Autodesk Fusion 360 part; units mm, degrees
sketch "Sketch1" plane through (0, 0, 0) normal (0, 0, 1) x (1, 0, 0)
  circle A0 centre (0, 0) radius 1.75
  circle A1 centre (0, 0) radius 5.25
  dimension "d1" = 3.5
  dimension "d2" = 3.5
extrude "Extrude1" add sketch "Sketch1" along normal blind 5
chamfer "Chamfer1" distance 1 angle 45 4 edges at (-1.6316, 0.6328, 5) (-4.8947, -1.8985, 5) (-4.8947, -1.8985, 0) (-1.6316, 0.6328, 0)
fillet "Fillet1" radius 1.25 4 edges at (-4.8947, -1.8985, 4) (-4.8947, 1.8985, 1) (-1.6316, 0.6328, 4) (-1.6316, -0.6328, 1)
fillet "Fillet2" radius 1.4 4 edges at (-3.9624, -1.5369, 0) (-2.5639, 0.9944, 0) (-2.5639, -0.9944, 5) (-3.9624, 1.5369, 5)
Geometry check sheet. Reference: the model listing, model coordinates, mm. Give positions to 0.01 mm unless a question says otherwise; leave off trailing zeros. Loops run counter-clockwise (first coordinate to the right, second up) from the corner with the lowest first, then second, coordinate; pieces in that order, holes last. Notation, with made-up numbers: M 64.25,65 L 85.25,65 A23 ccw 85.25,100 Z; hole C 26,39 d5. An arc over 180 degrees is marked long. Answer as a JSON object with one key per item and string values. Group by question number.
Item 1: Mould release check, pull along X, two halves, no side actions. Record for faces 1 (the cylindrical face through (1.617, 0.67, 2.486)), 2 (the cylindrical face through (5, -1.6, 2.5)): pulls with the +X half, pulls with the -X half, needs draft (parallel to the pull), parting line crosses it, or undercut.
Item 2: Gauge pin test, flat ends, axial feed: pin 1 (2 mm diameter, centred on x = 1.5, z = 2, fed in from -Y); pin 2 (2 mm diameter, centred on y = 4, z = 4, fed in from -X); pin 3 (1.5 mm diameter, centred on x = 2.5, z = 4, fed in from -Y). Record the tip position at first contact, or that the pin passes through.
Item 3: Material ranges on L1, parallel to Y at x = 0, z = 2.85; L2, parallel to X at y = -0.25, z = 3.75, recorded low to high.
Item 4: Sectioned sample at A-A on z = 2.45. Record the boundary of the cut face in (x, y), plus the area to 3 significant figures.
Findings below:
{
 "1": {"face 1": "undercut", "face 2": "parting line crosses it"},
 "2": {"pin 1": "y = -5.23", "pin 2": "x = -4.25", "pin 3": "y = -4.91"},
 "3": {"L1": "-5.25 to -1.75, 1.75 to 5.25", "L2": "-5.21 to -1.76, 1.76 to 5.21"},
 "4": {"outline": "C 0,0 d10.5; hole C 0,0 d3.5", "area": "77.0 mm2"}
}
